Geometry check sheet. Reference: the model listing, model coordinates, mm. A direction names the side the tool comes from. Coordinates: 2 decimals unless noted, no trailing zeros. Write each loop counter-clockwise with the first axis right and the second up, starting at its lowest first coordinate (ties: lowest second). Pieces come first, ordered by that corner, then holes. Notation, with made-up numbers: (-36, 10) -> (-20, 10) arc R31 cw to (-20, 44) -> close; hole circle Ø3 at (23, 60.25). An arc over 180 degrees is marked (long way). Answer in a Markdown table with one row per item. Add a question column.
1. Mould release check, pull along Y, two halves, no side actions. Record for faces 1 (the cylindrical face through (3.61, -8.8, -0.1)), 2 (the flat face through (2, 4.121, 0)), 3 (the flat face through (4.46, 9.73, 5.99)), 4 (the cylindrical face through (3.61, 8.8, 0.1)): pulls with the +Y half, pulls with the -Y half, needs draft (parallel to the pull), parting line crosses it, or undercut.
2. Cross-section at C-C on y = 8. Record the cut outline in (x, z).
3. Depth check by flat-ended pin: P1, Ø0.9, axis at x = 2.5, z = 1.5, coming from the +Y side; P2, Ø2, axis at x = -1.5, y = 4, coming from the -Z side; P3, Ø1.2, axis at y = -10, z = 3, coming from the -X side. Enter the tip coordinate at first touch or a pass-through.
4. Cross-section at D-D on z = 4.75. Record the cut outline in (x, y), and give its area (3 significant figures).
5. Scan lines: L1, parallel to X at y = 4.75, z = 5.75; L2, parallel to Z at x = -2.5, y = -4.5; L3, parallel to X at y = 7.5, z = 6.5. Record each from-to range of solid material in increasing order. Write a range as from..to.
6. Set-up check for faces 5 (the flat face through (-3.6, 1, 0)), 6 (the flat face through (4.44, -9.732, 6.006)), 7 (the flat face through (2, 8.5, 0)), 8 (the flat face through (2, -8.5, 0)): record each of +Z, -Z, +X, -X, +Y, -Y from which the full face is reachable in a straight line by a thin tool's end or side.
7. Cross-section at A-A on y = -1. Record the cut outline in (x, z).
8. Cross-section at B-B on z = -0.5. Record the cut outline in (x, y).
```python
from build123d import *

# Parameters (mm, degrees)
SKETCH1_W               = 7.5
SKETCH1_H               = 17
CUT_EXTRUDE1_START      = -20
CUT_EXTRUDE1_DEPTH      = 20
SKETCH4_W               = 1.6
SKETCH4_H               = 2
CUT_EXTRUDE2_DEPTH      = 20
CUT_EXTRUDE3_DEPTH      = 13.389511693
CUT_EXTRUDE3_DEPTH_BACK = 13.389511693
CUT_EXTRUDE4_DEPTH      = 13.389511863
CUT_EXTRUDE4_DEPTH_BACK = 13.389511863
BOSS_EXTRUDE4_DEPTH     = 2.5
FILLET1_R               = 1
BOSS_EXTRUDE7_DEPTH     = 2.5
FILLET5_R               = 1


with BuildPart() as part:
    # Sketch1 → Revolve1 (revolve)
    with BuildSketch(Plane.XY):
        with Locations((-3.75, 0)):
            Rectangle(SKETCH1_W, SKETCH1_H)
    revolve(axis=Axis((0, 8.5, 0), (0, -1, 0)))

    # Sketch2 → Cut-Extrude1 (cut)
    with BuildSketch(Plane.XZ.offset(8.5).offset(CUT_EXTRUDE1_START)):
        with BuildLine():
            Line((-5, 5.590169944), (-5, -5.590169944))
            ThreePointArc((-5, -5.590169944), (-7.5, 0), (-5, 5.590169944))
        make_face()
    cut_extrude1 = extrude(amount=CUT_EXTRUDE1_DEPTH, mode=Mode.SUBTRACT)

    # Sketch4 → Cut-Extrude2 (cut)
    with BuildSketch(Plane.XZ.offset(8.5)):
        with Locations((-2.8, 0)):
            Rectangle(SKETCH4_W, SKETCH4_H)
    extrude(amount=-CUT_EXTRUDE2_DEPTH, mode=Mode.SUBTRACT)

    # Mirror1: Cut-Extrude1 across plane
    add(cut_extrude1.mirror(Plane(origin=(0, 0, 0), x_dir=(0, 0, 1), z_dir=(1, 0, 0))), mode=Mode.SUBTRACT)

    # Sketch7 → Cut-Extrude3 (cut, two sides: drawn at the far end of the back side and taken through both)
    with BuildSketch(Plane.XY.offset(-CUT_EXTRUDE3_DEPTH_BACK)):
        with BuildLine():
            Line((0.441294084, 4.12121402), (2.641294084, 4.12121402))
            ThreePointArc((2.641294084, 4.12121402), (2.930486649, 4.17531345), (3.180566332, 4.330294869))
            ThreePointArc((3.180566332, 4.330294869), (3.374330031, 5.241617362), (2.573852958, 5.718366261))
            Line((2.573852958, 5.718366261), (1.796324142, 8.5))
            Line((1.796324142, 8.5), (-0.431632782, 8.5))
            Line((-0.431632782, 8.5), (0.38797004, 5.719434883))
            ThreePointArc((0.38797004, 5.719434883), (-0.156844774, 5.452467167), (-0.357641011, 4.879950081))
            ThreePointArc((-0.357641011, 4.879950081), (-0.109609196, 4.341123014), (0.441294084, 4.12121402))
        make_face()
    extrude(amount=CUT_EXTRUDE3_DEPTH + CUT_EXTRUDE3_DEPTH_BACK, mode=Mode.SUBTRACT)

    # Sketch8 → Cut-Extrude4 (cut, two sides: drawn at the far end of the back side and taken through both)
    with BuildSketch(Plane.XY.offset(-CUT_EXTRUDE4_DEPTH_BACK)):
        Polygon((-5, -5.268946984), (0.867668731, -8.5), (-5, -8.5), align=None)
    extrude(amount=CUT_EXTRUDE4_DEPTH + CUT_EXTRUDE4_DEPTH_BACK, mode=Mode.SUBTRACT)

    # Sketch13 → Boss-Extrude4 (add)
    with BuildSketch(Plane(origin=(0, 8.5, 0), x_dir=(1, 0, 0), z_dir=(0, 1, 0))):
        Polygon((5, 5.590169944), (5, -5.590169944), (3.894868524, -6.40936808), (3.894868524, 6.40936808), align=None)
    extrude(amount=BOSS_EXTRUDE4_DEPTH)

    # Fillet1
    # the kernel refuses this fillet: 1 mm, written as the material it adds along each edge
    with BuildSketch(Plane(origin=(3.894868524, 8.5, 8.90936808), x_dir=(-1, 0, 0), z_dir=(0, 0, -1))) as fillet1_piece_1_section:
        with BuildLine():
            CenterArc((FILLET1_R, FILLET1_R), FILLET1_R, 180, 90)
            Line((0, FILLET1_R), (0, 0))
            Line((0, 0), (FILLET1_R, 0))
        make_face()
    fillet1_piece_1 = extrude(amount=17.81873616, mode=Mode.PRIVATE)
    fillet1_piece_1 = fillet1_piece_1 & Plane(origin=(0, 8.724088474, 0), x_dir=(-1, 0, 0), z_dir=(0, 1, 0)) * Cylinder(7.5, 40, mode=Mode.PRIVATE)
    fillet1_piece_1 = split(fillet1_piece_1, bisect_by=Plane(origin=(6.812525482, 8.724088474, 4.246603564), z_dir=(-0.5955008037670206, -6.20137611558393e-15, -0.8033547116391566)), keep=Keep.TOP, mode=Mode.PRIVATE)
    add(fillet1_piece_1)

    # Sketch15 → Boss-Extrude7 (add)
    with BuildSketch(Plane.XZ.offset(8.5)):
        Polygon((5, 5.590169944), (5, -5.590169944), (3.894868524, -6.40936808), (3.894868524, 6.40936808), align=None)
    extrude(amount=BOSS_EXTRUDE7_DEPTH)

    # Fillet5
    # the kernel refuses this fillet: 1 mm, written as the material it adds along each edge
    with BuildSketch(Plane(origin=(3.894868524, -8.5, -8.90936808), x_dir=(-1, 0, 0), z_dir=(0, 0, 1))) as fillet5_piece_1_section:
        with BuildLine():
            CenterArc((FILLET5_R, FILLET5_R), FILLET5_R, 180, 90)
            Line((0, FILLET5_R), (0, 0))
            Line((0, 0), (FILLET5_R, 0))
        make_face()
    fillet5_piece_1 = extrude(amount=17.81873616, mode=Mode.PRIVATE)
    fillet5_piece_1 = fillet5_piece_1 & Plane(origin=(0, -8.724088474, 0), x_dir=(-1, 0, 0), z_dir=(0, 1, 0)) * Cylinder(7.5, 40, mode=Mode.PRIVATE)
    fillet5_piece_1 = split(fillet5_piece_1, bisect_by=Plane(origin=(6.812525482, -8.724088474, -4.246603564), z_dir=(-0.5955008037671681, -6.201376115585466e-15, 0.8033547116390474)), keep=Keep.TOP, mode=Mode.PRIVATE)
    add(fillet5_piece_1)


solid = part.part
```
Results found:
| question | item | result |
|---|---|---|
| 1 | face 1 | pulls with the -Y half |
| 1 | face 2 | undercut |
| 1 | face 3 | needs draft |
| 1 | face 4 | pulls with the +Y half |
| 2 | outline | (-5, -5.59) arc R7.5 ccw to (-0.28, -7.49) -> (-0.28, 7.49) arc R7.5 ccw to (-5, 5.59) -> close; (1.94, -7.25) arc R7.5 ccw to (5, -5.59) -> (5, 5.59) arc R7.5 ccw to (1.94, 7.25) -> close; hole (-3.6, -1) -> (-2, -1) -> (-2, 1) -> (-3.6, 1) -> close |
| 3 | P1 | stops at y = 8.5 |
| 3 | P2 | stops at z = -7.48 |
| 3 | P3 | stops at x = 3.89 |
| 4 | outline | (-5, -5.27) -> (0.87, -8.5) -> (2.89, -8.5) arc R1 cw to (3.89, -9.5) -> (3.89, -11) -> (5, -11) -> (5, 11) -> (3.89, 11) -> (3.89, 9.5) arc R1 cw to (2.89, 8.5) -> (1.8, 8.5) -> (2.57, 5.72) arc R0.8 cw (long way) to (2.64, 4.12) -> (0.44, 4.12) arc R0.8 cw to (0.39, 5.72) -> (-0.43, 8.5) -> (-5, 8.5) -> close |
| 4 | area | 155 mm^2 |
| 5 | L1 | x = -4.82..-0.34, 3.42..4.82 |
| 5 | L2 | z = -7.07..-1, 1..7.07 |
| 5 | L3 | x = -3.74..-0.14, 2.08..3.74 |
| 6 | face 5 | +Y, -Y |
| 6 | face 6 | +Z, +X, -Y |
| 6 | face 7 | +Z, -Z, -X, +Y |
| 6 | face 8 | +Z, -Z, -X, -Y |
| 7 | outline | (-5, -5.59) arc R7.5 ccw to (5, -5.59) -> (5, 5.59) arc R7.5 ccw to (-5, 5.59) -> close; hole (-3.6, -1) -> (-2, -1) -> (-2, 1) -> (-3.6, 1) -> close |
| 8 | outline | (-5, -5.27) -> (-3.6, -6.04) -> (-3.6, 8.5) -> (-5, 8.5) -> close; (-2, -6.92) -> (0.87, -8.5) -> (2.89, -8.5) arc R1 cw to (3.89, -9.5) -> (3.89, -11) -> (5, -11) -> (5, 11) -> (3.89, 11) -> (3.89, 9.5) arc R1 cw to (2.89, 8.5) -> (1.8, 8.5) -> (2.57, 5.72) arc R0.8 cw (long way) to (2.64, 4.12) -> (0.44, 4.12) arc R0.8 cw to (0.39, 5.72) -> (-0.43, 8.5) -> (-2, 8.5) -> close |
